Model file for the job. Use its own axes, mm. Face numbers are marked on the shaded views. A direction names the side the tool comes from. Coordinates: 2 decimals unless noted, no trailing zeros. Write each loop counter-clockwise with the first axis right and the second up, starting at its lowest first coordinate (ties: lowest second). Pieces come first, ordered by that corner, then holes.
Q1. Drill centre lines: probe 1 along Y at (x, z) = (-17.5, 2.5); probe 2 along X at (y, z) = (-7, 5); probe 3 along X at (y, z) = (-4, 4.5). Where is each one in solid material? Low to high.
Q2. Pull direction Z, two halves, no side cores. Call the marked faces 6, 7, 8 and 9: released by +Z, released by -Z, zero draft, split by the parting line, or undercut.
Q3. Band-saw the part on A-A, the plane y = 9. Write the cut outline in (x, z).
Q4. Pin check, flat tips, straight feed: P1, Ø3, axis at y = 6, z = 9.5, coming from the +X side; P2, Ø1.9, axis at x = -15.5, z = 9.5, coming from the -Y side; P3, Ø5, axis at x = -10, z = 4.5, coming from the +Y side. Stop position of each tip, or through.
Q5. Band-saw the part on D-D, the plane y = -8. Write the cut outline in (x, z).
Q6. Band-saw the part on B-B, the plane x = 11.5. Write the cut outline in (y, z).
Q7. Which spindle directions (+Z, -Z, +X, -X, +Y, -Y) get a long thin tool onto all of the face, cutting with end or side? Do the marked faces 1, 2, 3, 4 and 5. Say none if no direction does.
Q8. Band-saw the part on C-C, the plane z = 13. Write the cut outline in (x, y).
from build123d import *

# Parameters (mm, degrees)
BOSS_EXTRUDE1_DEPTH = 13.716
SKETCH2_R           = 5.4864
CUT_EXTRUDE1_DEPTH  = 3.6068
SKETCH3_R           = 2.921
CUT_EXTRUDE2_DEPTH  = 27.267149632
FILLET1_R           = 0.127
FILLET2_R           = 0.127
FILLET3_R           = 1.27
FILLET4_R           = 0.127


with BuildPart() as part:
    # Sketch1 → Boss-Extrude1 (new body)
    with BuildSketch(Plane.XY):
        with BuildLine():
            Line((-18.286658229, -2.8956), (-14.409782184, -2.8956))
            ThreePointArc((-14.409782184, -2.8956), (-13.697921632, -3.607460552), (-12.986061079, -2.8956))
            Line((-12.986061079, -2.8956), (-9.224054916, -2.8956))
            ThreePointArc((-9.224054916, -2.8956), (-8.450188338, -3.158609176), (-7.996847762, -3.838701544))
            ThreePointArc((-7.996847762, -3.838701544), (9.003275389, -14.686851959), (21.268740456, 1.3208))
            ThreePointArc((21.268740456, 1.3208), (7.692360315, 14.858458112), (-7.996847762, 3.838701544))
            ThreePointArc((-7.996847762, 3.838701544), (-8.450188338, 3.158609176), (-9.224054916, 2.8956))
            Line((-9.224054916, 2.8956), (-12.986061079, 2.8956))
            ThreePointArc((-12.986061079, 2.8956), (-13.697921632, 3.607460552), (-14.409782184, 2.8956))
            Line((-14.409782184, 2.8956), (-18.286658229, 2.8956))
            ThreePointArc((-18.286658229, 2.8956), (-18.958421102, 3.087808442), (-19.426847762, 3.606254106))
            Line((-19.426847762, 3.606254106), (-19.426847762, 11.2776))
            ThreePointArc((-19.426847762, 11.2776), (-19.054873374, 12.175625612), (-18.156847762, 12.5476))
            Line((-18.156847762, 12.5476), (-6.510253262, 12.5476))
            ThreePointArc((-6.510253262, 12.5476), (-5.629373118, 12.705237691), (-4.857831488, 13.158584116))
            ThreePointArc((-4.857831488, 13.158584116), (13.050680986, 16.004898652), (23.689927776, 1.3208))
            ThreePointArc((23.689927776, 1.3208), (14.251434441, -15.452408322), (-4.857831488, -13.158584116))
            ThreePointArc((-4.857831488, -13.158584116), (-5.629373118, -12.705237691), (-6.510253262, -12.5476))
            Line((-6.510253262, -12.5476), (-18.156847762, -12.5476))
            ThreePointArc((-18.156847762, -12.5476), (-19.054873374, -12.175625612), (-19.426847762, -11.2776))
            Line((-19.426847762, -11.2776), (-19.426847762, -3.606254106))
            ThreePointArc((-19.426847762, -3.606254106), (-18.958421102, -3.087808442), (-18.286658229, -2.8956))
        make_face()
    extrude(amount=BOSS_EXTRUDE1_DEPTH)

    # Sketch2 → Cut-Extrude1 (cut)
    with BuildSketch(Plane.XZ.offset(12.5476)):
        with Locations((-12.333550512, 6.858)):
            Circle(SKETCH2_R)
    extrude(amount=-CUT_EXTRUDE1_DEPTH, mode=Mode.SUBTRACT)

    # Sketch3 → Cut-Extrude2 (cut, through all)
    with BuildSketch(Plane.XZ.offset(8.9408)):
        with Locations((-12.333550512, 6.858)):
            Circle(SKETCH3_R)
    extrude(amount=-CUT_EXTRUDE2_DEPTH, mode=Mode.SUBTRACT)

    # Fillet1
    fillet1_edges = [part.edges().sort_by_distance(p)[0] for p in [
        (-15.254550512, 12.5476, 6.858),
    ]]
    fillet(fillet1_edges, radius=FILLET1_R)

    # Fillet2
    fillet2_edges = [part.edges().sort_by_distance(p)[0] for p in [
        (-17.819950512, -12.5476, 6.858),
    ]]
    fillet(fillet2_edges, radius=FILLET2_R)

    # Fillet3
    fillet3_edges = [part.edges().sort_by_distance(p)[0] for p in [
        (-17.819950512, -8.9408, 6.858),
    ]]
    fillet(fillet3_edges, radius=FILLET3_R)

    # Fillet4
    fillet4_edges = [part.edges().sort_by_distance(p)[0] for p in [
        (-15.254550512, -8.9408, 6.858),
    ]]
    fillet(fillet4_edges, radius=FILLET4_R)


solid = part.part
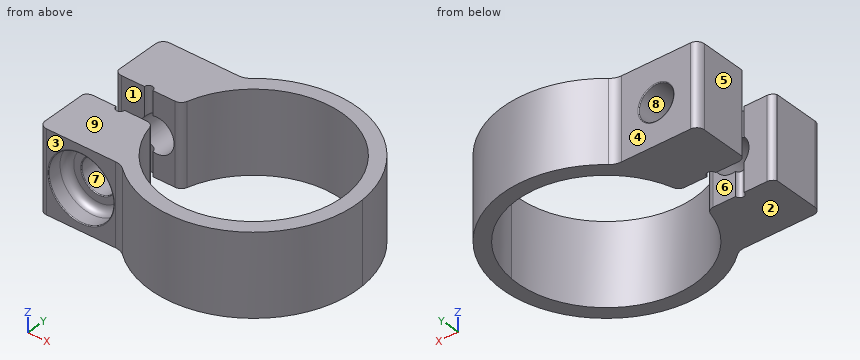
Answer sheet:
1. probe 1: y = -12.55 to -2.9, 2.9 to 12.55
1. probe 2: x = -19.43 to -14.59, -10.08 to -6.75, 19.58 to 22.26
1. probe 3: x = -19.43 to -14.06, -10.61 to -7.95, 20.78 to 23.27
2. face 6: zero draft
2. face 7: undercut
2. face 8: undercut
2. face 9: released by +Z
3. outline: (-19.43, 0) - (-5.48, 0) - (-5.48, 13.72) - (-19.43, 13.72) - close; (18.31, 0) - (21.22, 0) - (21.22, 13.72) - (18.31, 13.72) - close; hole circle Ø5.84 at (-12.33, 6.86)
4. P1: stops at x = 23.15
4. P2: stops at y = -9.27
4. P3: stops at y = 12.55
5. outline: (-19.43, 0) - (-6.17, 0) - (-6.17, 13.72) - (-19.43, 13.72) - close; (19, 0) - (21.78, 0) - (21.78, 13.72) - (19, 13.72) - close; hole circle Ø5.84 at (-12.33, 6.86)
6. outline: (-16.56, 0) - (-14.02, 0) - (-14.02, 13.72) - (-16.56, 13.72) - close; (14.02, 0) - (16.56, 0) - (16.56, 13.72) - (14.02, 13.72) - close
7. face 1: +Z, -Z, -X
7. face 2: -Z, +X, -X, +Y, -Y
7. face 3: +Z, -Z, -X, -Y
7. face 4: +Z, -Z, -X, +Y
7. face 5: +Z, -Z, -X, +Y, -Y
8. outline: (-19.43, -11.28) arc R1.27 ccw to (-18.16, -12.55) - (-6.51, -12.55) arc R2.54 cw to (-4.86, -13.16) arc R17.33 ccw (long way) to (-4.86, 13.16) arc R2.54 cw to (-6.51, 12.55) - (-18.16, 12.55) arc R1.27 ccw to (-19.43, 11.28) - (-19.43, 3.61) arc R1.27 ccw to (-18.29, 2.9) - (-14.41, 2.9) arc R0.71 cw to (-12.99, 2.9) - (-9.22, 2.9) arc R1.27 ccw to (-8, 3.84) arc R14.91 cw (long way) to (-8, -3.84) arc R1.27 ccw to (-9.22, -2.9) - (-12.99, -2.9) arc R0.71 cw to (-14.41, -2.9) - (-18.29, -2.9) arc R1.27 ccw to (-19.43, -3.61) - close
